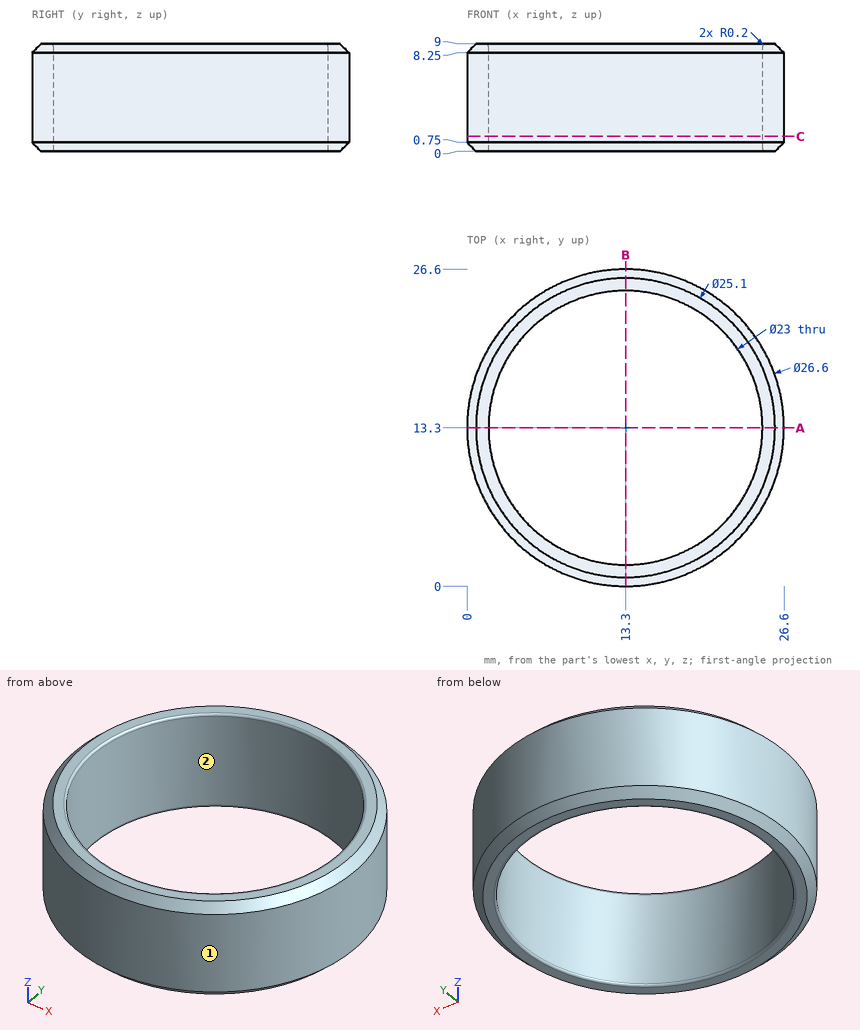
Can you work these out from the drawing? Everything is in mm from the part's minimum corner. Round coordinates to 2 decimals unless told otherwise and drop trailing zeros. Write each loop counter-clockwise with the first axis right and the second up, starting at its lowest first coordinate (ties: lowest second). Pieces come first, ordered by that corner, then holes. Notation, with made-up numbers: (-21, 64.25) - (28, 64.25) arc R22 cw to (28, 89.25) - close; hole circle Ø5 at (5, 64). An arc over 180 degrees is marked (long way). Put each result on its own line as item: value. Start each with the question number.
(1) Will these pins go through, and if not, where does the flat tip stop? pin 1 (12 mm diameter, centred on x = 19.5, y = 3, fed in from -Z); pin 2 (1 mm diameter, centred on x = 21.5, z = 4.5, fed in from -Y); pin 3 (1.5 mm diameter, centred on x = 18, z = 7, fed in from -Y); pin 4 (1 mm diameter, centred on x = 19.5, z = 4.5, fed in from -Y).
(2) Thinking about a two-plate mould opening in Y: for the marked faces 1 and 2, which applies, released by +Y, released by -Y, zero draft, split by the parting line, or undercut?
(3) I want a section at A-A, the plane y = 13.3. Please give me the cut outline in (x, z).
(4) I need wall thicknesses on probe 1 along Y at (x, z) = (13.3, 5.5); probe 2 along Y at (x, z) = (10.75, 7.5); probe 3 along X at (y, z) = (19.5, 2.5). Which ranges of each line are inside material? Lowest first, please.
(5) I want a section at C-C, the plane z = 1.25. Please give me the cut outline in (x, y).
Here are the results:
1. pin 1: stops at z = 0
1. pin 2: stops at y = 2.46
1. pin 3: stops at y = 0.6
1. pin 4: stops at y = 1.28
2. face 1: split by the parting line
2. face 2: undercut
3. outline: (0, 0.75) - (0.75, 0) - (1.6, 0) arc R0.2 ccw to (1.8, 0.2) - (1.8, 8.8) arc R0.2 ccw to (1.6, 9) - (0.75, 9) - (0, 8.25) - close; (24.8, 0.2) arc R0.2 ccw to (25, 0) - (25.85, 0) - (26.6, 0.75) - (26.6, 8.25) - (25.85, 9) - (25, 9) arc R0.2 ccw to (24.8, 8.8) - close
4. probe 1: y = 0 to 1.8, 24.8 to 26.6
4. probe 2: y = 0.25 to 2.09, 24.51 to 26.35
4. probe 3: x = 1.53 to 3.61, 22.99 to 25.07
5. outline: circle Ø26.6 at (13.3, 13.3); hole circle Ø23 at (13.3, 13.3)
